Verification items for the finished model (mm, model axes). A direction names the side the tool comes from. Coordinates: 2 decimals unless noted, no trailing zeros. Write each loop counter-clockwise with the first axis right and the second up, starting at its lowest first coordinate (ties: lowest second). Pieces come first, ordered by that corner, then holes. Notation, with made-up numbers: M -29,-33.75 L 2,-33.75 A33 cw 2,-0.75 Z; hole C -33,-15 d6. An arc over 180 degrees is marked long. One line per item, written item: value.
```python
from build123d import *

# Parameters (mm, degrees)
F0_R     = 1.65
F1_DEPTH = 6
F2_DEPTH = 5
F4_R     = 2
F3_R     = 1.3
F5_DEPTH = 7
F3_R_2   = 1.55
F6_DEPTH = 3
F7_R     = 1


with BuildPart() as f1:
    # F0 (on Top) → F1 (new body)
    with BuildSketch(Plane.XY):
        with BuildLine():
            Line((1.18, 0), (0, 0))
            Line((0, 0), (-1.18, 0))
            Line((-1.18, 0), (-1.18, 7))
            Line((-1.18, 7), (-3.18, 7))
            Line((-3.18, 7), (-3.18, 0))
            Line((-3.18, 0), (-3.18, -3))
            Line((-3.18, -3), (-18.18, -3))
            ThreePointArc((-18.18, -3), (-20.3013203436, -3.8786796564), (-21.18, -6))
            Line((-21.18, -6), (-21.18, -12))
            Line((-21.18, -12), (-19.68, -12))
            Line((-19.68, -12), (-19.68, -6))
            ThreePointArc((-19.68, -6), (-19.2406601718, -4.9393398282), (-18.18, -4.5))
            Line((-18.18, -4.5), (-12.78, -4.5))
            Line((-12.78, -4.5), (0, -4.5))
            Line((0, -4.5), (12.78, -4.5))
            Line((12.78, -4.5), (18.18, -4.5))
            ThreePointArc((18.18, -4.5), (19.2406601718, -4.9393398282), (19.68, -6))
            Line((19.68, -6), (19.68, -12))
            Line((19.68, -12), (21.18, -12))
            Line((21.18, -12), (21.18, -6))
            ThreePointArc((21.18, -6), (20.3013203436, -3.8786796564), (18.18, -3))
            Line((18.18, -3), (3.18, -3))
            Line((3.18, -3), (3.18, 0))
            Line((3.18, 0), (3.18, 7))
            Line((3.18, 7), (1.18, 7))
            Line((1.18, 7), (1.18, 0))
        make_face()
        with BuildLine():
            Line((15.78, -12), (19.68, -12))
            Line((19.68, -12), (19.68, -6))
            ThreePointArc((19.68, -6), (19.2406601718, -4.9393398282), (18.18, -4.5))
            Line((18.18, -4.5), (12.78, -4.5))
            Line((12.78, -4.5), (12.78, -9))
            ThreePointArc((12.78, -9), (13.6586796564, -11.1213203436), (15.78, -12))
        make_face()
        with Locations((16.43, -8.35)):
            Circle(F0_R, mode=Mode.SUBTRACT)
        with BuildLine():
            Line((-19.68, -6), (-19.68, -12))
            Line((-19.68, -12), (-15.78, -12))
            ThreePointArc((-15.78, -12), (-13.6586796564, -11.1213203436), (-12.78, -9))
            Line((-12.78, -9), (-12.78, -4.5))
            Line((-12.78, -4.5), (-18.18, -4.5))
            ThreePointArc((-18.18, -4.5), (-19.2406601718, -4.9393398282), (-19.68, -6))
        make_face()
        with Locations((-16.43, -8.35)):
            Circle(F0_R, mode=Mode.SUBTRACT)
    extrude(amount=F1_DEPTH)

    # F0 (on Top) → F2 (cut)
    with BuildSketch(Plane.XY):
        with BuildLine():
            Line((-19.68, -6), (-19.68, -12))
            Line((-19.68, -12), (-15.78, -12))
            ThreePointArc((-15.78, -12), (-13.6586796564, -11.1213203436), (-12.78, -9))
            Line((-12.78, -9), (-12.78, -4.5))
            Line((-12.78, -4.5), (-18.18, -4.5))
            ThreePointArc((-18.18, -4.5), (-19.2406601718, -4.9393398282), (-19.68, -6))
        make_face()
        with Locations((-16.43, -8.35)):
            Circle(F0_R, mode=Mode.SUBTRACT)
        with BuildLine():
            Line((15.78, -12), (19.68, -12))
            Line((19.68, -12), (19.68, -6))
            ThreePointArc((19.68, -6), (19.2406601718, -4.9393398282), (18.18, -4.5))
            Line((18.18, -4.5), (12.78, -4.5))
            Line((12.78, -4.5), (12.78, -9))
            ThreePointArc((12.78, -9), (13.6586796564, -11.1213203436), (15.78, -12))
        make_face()
        with Locations((16.43, -8.35)):
            Circle(F0_R, mode=Mode.SUBTRACT)
    extrude(amount=F2_DEPTH, mode=Mode.SUBTRACT)

    # F4
    f4_edges = [f1.edges().sort_by_distance(p)[0] for p in [
        (-2.18, 7, 6),
        (2.18, 7, 6),
        (2.18, 7, 0),
        (-2.18, 7, 0),
    ]]
    fillet(f4_edges, radius=F4_R)

    # F3 (on face) → F5 (cut)
    with BuildSketch(Plane(origin=(-3.18, 0, 0), x_dir=(0, -1, 0), z_dir=(-1, 0, 0))):
        with Locations((-3.45, 3.0407507438)):
            Circle(F3_R)
    extrude(amount=-F5_DEPTH, mode=Mode.SUBTRACT)

    # F3 (on face) → F6 (cut)
    with BuildSketch(Plane(origin=(-3.18, 0, 0), x_dir=(0, -1, 0), z_dir=(-1, 0, 0))):
        with Locations((-3.45, 3.0407507438)):
            Circle(F3_R_2)
        with Locations((-3.45, 3.0407507438)):
            Circle(F3_R, mode=Mode.SUBTRACT)
    extrude(amount=-F6_DEPTH, mode=Mode.SUBTRACT)

    # F7
    f7_edges = [f1.edges().sort_by_distance(p)[0] for p in [
        (-19.68, -9, 5),
        (15.48, -4.5, 5),
        (12.78, -4.5, 5.5),
        (-12.78, -4.5, 5.5),
        (-20.43, -12, 0),
        (20.43, -12, 0),
        (3.18, -3, 3),
        (-3.18, -3, 3),
        (0, 0, 6),
        (0, 0, 0),
    ]]
    fillet(f7_edges, radius=F7_R)


solid = f1.part
```
Item 1: Cross-section at A-A, the plane x = -16.43. Enter the section's corners in (y, z), and give its area (3 significant figures).
The answers:
outline: M -12,5 L -10,5 L -10,6 L -12,6 Z; M -6.7,5 L -5.5,5 A1 cw -4.5,4 L -4.5,0 L -3,0 L -3,6 L -6.7,6 Z
area: 13.4 mm²
Item 2: Cross-section at B-B, the plane y = 3.45. Enter the section's corners in (x, z), and give its area (3 significant figures).
The answers:
outline: M -3.18,0 L -1.18,0 L -1.18,1.49 L -3.18,1.49 Z; M -3.18,4.59 L -1.18,4.59 L -1.18,6 L -3.18,6 Z; M 1.18,0 L 3.18,0 L 3.18,1.74 L 1.18,1.74 Z; M 1.18,4.34 L 3.18,4.34 L 3.18,6 L 1.18,6 Z
area: 12.6 mm²
Item 3: Access from +Z, -Z, +X, -X, +Y, -Y to the whole of each face (thin tool, end or side, straight path). Record for faces 4 (the face through (3.18, 1, 3)), 5 (the face through (-12.34, -4.67, 5.24)), 6 (the face through (-2.19, 6.4, 5.43)), 7 (the face through (19.395, -8.958, 4.699)).
The answers:
face 4: +Z, -Z, +X, +Y
face 5: +Z, -Z, -Y
face 6: +Z, +X, -X, +Y
face 7: -Z, -Y
Item 4: Go/stop test with flat-tipped pins: P1, Ø3, axis at y = -2, z = 3.5, coming from the +X side; P2, Ø1.2, axis at x = 0.5, z = 2.5, coming from the +Y side; P3, Ø1.8, axis at x = -12, z = 3, coming from the +Y side. Record where each tip stops, or that it passes through.
The answers:
P1: stops at x = 19.84
P2: stops at y = 0
P3: stops at y = -3
Item 5: Cross-section at C-C, the plane x = -7.5. Enter the section's corners in (y, z), and give its area (3 significant figures).
The answers:
outline: M -4.5,0 L -3,0 L -3,6 L -4.5,6 Z
area: 9.00 mm²
Item 6: Draft check along X on faces 1 (the face through (21.18, -9, 3)), 2 (the face through (2.17, 4.48, 2.25)), 3 (the face through (0, 0, 3)). Enter one of: released by +X, released by -X, zero draft, split by the parting line, or undercut.
The answers:
face 1: released by +X
face 2: zero draft
face 3: undercut
Item 7: Scan lines: line 1 (Y direction, x = 16.43, z = 5.7); line 2 (X direction, y = 5.25, z = 0.95); line 3 (X direction, y = -9.75, z = 3.1). Record each from-to range of solid material in increasing order.
The answers:
line 1: y = -12 to -10, -6.7 to -3
line 2: x = -3.18 to -1.18, 1.18 to 3.18
line 3: x = -21.18 to -19.68, 19.68 to 21.18
